Build history of the part. All positions in model axes, mm. A direction names the side the tool comes from. Round coordinates to 2 decimals unless told otherwise and drop trailing zeros. Order: outer loops, then holes, each group sorted by start corner. A loop starts at its lowest first (then second) coordinate and runs counter-clockwise, first axis right, second up. Notation, with made-up numbers: (80.5, 5.5) - (102.5, 5.5) arc R30 ccw to (102.5, 34.5) - close; hole circle Ø5 at (22, 23.5). An arc over 180 degrees is marked (long way). One line per question, with ' | ' between items. Start each with the question number.
from build123d import *

# Parameters (mm, degrees)
SKETCH_W        = 41.2
SKETCH_H        = 101.6
PAD_DEPTH       = 1.6
SKETCH001_W     = 1.2
SKETCH001_H     = 101.6
PAD001_DEPTH    = 11.6
SKETCH002_W     = 41.2
SKETCH002_H     = 13.2
PAD002_DEPTH    = 1.6
SKETCH003_W     = 30
SKETCH003_H     = 11.2
POCKET_DEPTH    = 1.2
SKETCH004_R     = 3
POCKET001_DEPTH = 1.6


with BuildPart() as part:
    # Sketch → Pad (new body)
    with BuildSketch(Plane.XY):
        with Locations((20.6, -50.8)):
            Rectangle(SKETCH_W, SKETCH_H)
    extrude(amount=PAD_DEPTH)

    # Sketch001 → Pad001 (new body)
    with BuildSketch(Plane.XY.offset(1.6)):
        with Locations((0.6, -50.8)):
            Rectangle(SKETCH001_W, SKETCH001_H)
        with Locations((40.6, -50.8)):
            Rectangle(SKETCH001_W, SKETCH001_H)
    extrude(amount=PAD001_DEPTH)

    # Sketch002 → Pad002 (new body)
    with BuildSketch(Plane.XZ.offset(101.6)):
        with Locations((20.6, 6.6)):
            Rectangle(SKETCH002_W, SKETCH002_H)
    extrude(amount=PAD002_DEPTH)

    # Sketch003 → Pocket (cut)
    with BuildSketch(Plane.YZ.offset(41.2)):
        with Locations((-51, 7.6)):
            Rectangle(SKETCH003_W, SKETCH003_H)
    extrude(amount=-POCKET_DEPTH, mode=Mode.SUBTRACT)

    # Sketch004 → Pocket001 (cut)
    with BuildSketch(Plane(origin=(0, 0, 0), x_dir=(1, 0, 0), z_dir=(0, 0, -1))):
        with Locations((32.7, 94.2)):
            Circle(SKETCH004_R)
        with Locations((9, 34.7)):
            Circle(SKETCH004_R)
        with Locations((32.7, 34.7)):
            Circle(SKETCH004_R)
    extrude(amount=-POCKET001_DEPTH, mode=Mode.SUBTRACT)


solid = part.part
Item 1: Slice it at C-C (y = -34.7). Write the cut outline in (x, z).
Item 2: Slice it at D-D (z = 4). Write the cut outline in (x, y), plus the area to 3 significant figures.
Item 3: Slice it at A-A (x = 32.7). Write the cut outline in (y, z).
Item 4: Slice it at B-B (x = 9). Write the cut outline in (y, z).
Item 5: 3-axis set-ups, long thin cutter, end or side, ignore diameter. For faces 4 (the face through (20, -101.6, 7)), 5 (the face through (30.49, -96.23, 0.79)): which of +Z, -Z, +X, -X, +Y, -Y reach the whole face in a straight line?
Item 6: Pin check, flat tips, straight feed: pin 1 (5 mm diameter, centred on y = -28, z = 7, fed in from -X); pin 2 (12 mm diameter, centred on x = 8, y = -63, fed in from +Z); pin 3 (1 mm diameter, centred on x = 40.5, y = -49, fed in from +Z); pin 4 (3.5 mm diameter, centred on x = 22.5, z = 6.5, fed in from +Y). Stop position of each tip, or through.
Item 7: Wall check: line 1 along Y through (x, z) = (32.7, 0.95); line 2 along Y through (x, z) = (9, 0.65); line 3 along X through (y, z) = (-31.5, 5.75). Give the ranges that are in metal, low to high. Write a range as [from, to].
Item 8: Pull direction X, two halves, no side cores. Call faces 1 (the face through (41.2, -51, 1)), 2 (the face through (1, -59, 13.2)), 3 (the face through (20, -50, 1.6)): released by +X, released by -X, zero draft, split by the parting line, or undercut.
A:
1) outline: (0, 0) - (6, 0) - (6, 1.6) - (1.2, 1.6) - (1.2, 13.2) - (0, 13.2) - close; (12, 0) - (29.7, 0) - (29.7, 1.6) - (12, 1.6) - close; (35.7, 0) - (41.2, 0) - (41.2, 13.2) - (40, 13.2) - (40, 1.6) - (35.7, 1.6) - close
2) outline: (0, -103.2) - (41.2, -103.2) - (41.2, -66) - (40, -66) - (40, -101.6) - (1.2, -101.6) - (1.2, 0) - (0, 0) - close; (40, -36) - (41.2, -36) - (41.2, 0) - (40, 0) - close | area: 274 mm^2
3) outline: (-103.2, 0) - (-97.2, 0) - (-97.2, 1.6) - (-101.6, 1.6) - (-101.6, 13.2) - (-103.2, 13.2) - close; (-91.2, 0) - (-37.7, 0) - (-37.7, 1.6) - (-91.2, 1.6) - close; (-31.7, 0) - (0, 0) - (0, 1.6) - (-31.7, 1.6) - close
4) outline: (-103.2, 0) - (-37.7, 0) - (-37.7, 1.6) - (-101.6, 1.6) - (-101.6, 13.2) - (-103.2, 13.2) - close; (-31.7, 0) - (0, 0) - (0, 1.6) - (-31.7, 1.6) - close
5) face 4: +Z, +Y | face 5: +Z, -Z
6) pin 1: x = 0 | pin 2: z = 1.6 | pin 3: z = 2 | pin 4: y = -101.6
7) line 1: [-103.2, -97.2], [-91.2, -37.7], [-31.7, 0] | line 2: [-103.2, -37.7], [-31.7, 0] | line 3: [0, 1.2], [40, 41.2]
8) face 1: released by +X | face 2: zero draft | face 3: undercut
